```python
from build123d import *

# Parameters (mm, degrees)
SKETCH2_W                = 114.356575713
SKETCH2_H                = 12.768326156
SKETCH2_R                = 3.048
BOSS_EXTRUDE1_DEPTH      = 3.81
BOSS_EXTRUDE2_DEPTH      = 3.81
BOSS_EXTRUDE2_DEPTH_BACK = 3.81


with BuildPart() as part:
    # Sketch2 → Boss-Extrude1 (new body)
    with BuildSketch(Plane.XY):
        with Locations((-0.028287857, -0.034163078)):
            Rectangle(SKETCH2_W, SKETCH2_H)
        with Locations((-46.99, 0)):
            Circle(SKETCH2_R, mode=Mode.SUBTRACT)
        with Locations((46.99, 0)):
            Circle(SKETCH2_R, mode=Mode.SUBTRACT)
    extrude(amount=BOSS_EXTRUDE1_DEPTH)

    # Sketch3 → Boss-Extrude2 (add, two sides)
    with BuildSketch(Plane(origin=(0, 0, 0), x_dir=(1, 0, 0), z_dir=(0, 1, 0))) as boss_extrude2_sk:
        with BuildLine():
            Line((0, 0), (22.86, 0))
            Line((22.86, 0), (22.86, 10.986323502))
            ThreePointArc((22.86, 10.986323502), (0, 1.27), (-22.86, 10.986323502))
            Line((-22.86, 10.986323502), (-22.86, 0))
            Line((-22.86, 0), (0, 0))
        make_face()
    extrude(amount=BOSS_EXTRUDE2_DEPTH)
    extrude(boss_extrude2_sk.sketch, amount=-BOSS_EXTRUDE2_DEPTH_BACK)


solid = part.part
```
Input: part model. Units: mm. Frame: model coordinates. A direction names the side the tool comes from. Round coordinates to 2 decimals unless told otherwise and drop trailing zeros. Loops run counter-clockwise (first coordinate to the right, second up) from the corner with the lowest first, then second, coordinate; pieces in that order, holes last. Notation, with made-up numbers: M 58,64 L 117,64 A21 cw 117,103 Z; hole C 16,-25.75 d7. An arc over 180 degrees is marked long. Answer in a Markdown table with one row per item. Add a question column.
1. Ray query, probe 1 along Y at (x, z) = (-46.99, 2.9); probe 2 along Z at (x, y) = (-31, -5); probe 3 along X at (y, z) = (3.75, -9.5). Return the intervals inside material, ascending.
2. Mould query, pull axis X, two halves, no side actions, for faces 1 (the face through (-57.207, 0, 2)), 2 (the face through (0.357, 0.053, -1.272)), 3 (the face through (0, 3.81, -1)), 4 (the face through (49.897, 0.916, 1.878)). Classes: released by +X, released by -X, zero draft, split by the parting line, or undercut.
3. Section B-B (y = 0). Output: boundary loops of the cut face in (x, z).
4. Contact query for flat-ended pins moving along their axis: pin 1 (2.5 mm diameter, centred on y = -1, z = -6, fed in from +X); pin 2 (4 mm diameter, centred on y = -1.5, z = -8.5, fed in from -X); pin 3 (1.5 mm diameter, centred on x = 14.5, z = -5.5, fed in from +Y); pin 4 (6 mm diameter, centred on y = -4, z = -1, fed in from +X). Output: stop coordinate, or through.
5. Section C-C (z = -7.5). Output: boundary loops of the cut face in (x, y), and give its area (3 significant figures).
6. Section A-A (x = 46.99). Output: boundary loops of the cut face in (y, z), and give its area (3 significant figures).
7. Set-up query: faces 5 (the face through (57.15, 0, 2)), 6 (the face through (22.86, 0, -5)), 7 (the face through (0, -3.81, -1)), 8 (the face through (-22.86, 0, -6)), 9 (the face through (-1, -6.418, 2)). Return all of +Z, -Z, +X, -X, +Y, -Y with unobstructed straight access to the full face (end or side cutting, diameter ignored); none if empty.
8. Section D-D (x = 5). Output: boundary loops of the cut face in (y, z), and give its area (3 significant figures).
Values follow:
| question | item | result |
|---|---|---|
| 1 | probe 1 | -6.42 to -3.05, 3.05 to 6.35 |
| 1 | probe 2 | 0 to 3.81 |
| 1 | probe 3 | -22.86 to -21.33, 21.33 to 22.86 |
| 2 | face 1 | released by -X |
| 2 | face 2 | undercut |
| 2 | face 3 | zero draft |
| 2 | face 4 | undercut |
| 3 | outline | M -57.21,0 L -50.04,0 L -50.04,3.81 L -57.21,3.81 Z; M -43.94,0 L -22.86,0 L -22.86,-10.99 A31.75 cw 22.86,-10.99 L 22.86,0 L 43.94,0 L 43.94,3.81 L -43.94,3.81 Z; M 50.04,0 L 57.15,0 L 57.15,3.81 L 50.04,3.81 Z |
| 4 | pin 1 | x = 22.86 |
| 4 | pin 2 | x = -22.86 |
| 4 | pin 3 | y = 3.81 |
| 4 | pin 4 | x = 57.15 |
| 5 | outline | M -22.86,-3.81 L -18.89,-3.81 L -18.89,3.81 L -22.86,3.81 Z; M 18.89,-3.81 L 22.86,-3.81 L 22.86,3.81 L 18.89,3.81 Z |
| 5 | area | 60.5 mm^2 |
| 6 | outline | M -6.42,0 L -3.05,0 L -3.05,3.81 L -6.42,3.81 Z; M 3.05,0 L 6.35,0 L 6.35,3.81 L 3.05,3.81 Z |
| 6 | area | 25.4 mm^2 |
| 7 | face 5 | +Z, -Z, +X, +Y, -Y |
| 7 | face 6 | -Z, +X, +Y, -Y |
| 7 | face 7 | -Z, +X, -X, -Y |
| 7 | face 8 | -Z, -X, +Y, -Y |
| 7 | face 9 | +Z, -Z, +X, -X, -Y |
| 8 | outline | M -6.42,0 L -3.81,0 L -3.81,-1.67 L 3.81,-1.67 L 3.81,0 L 6.35,0 L 6.35,3.81 L -6.42,3.81 Z |
| 8 | area | 61.3 mm^2 |
